Could you check a few things on this model? Use its own coordinates, in mm. Round coordinates to 2 decimals unless told otherwise and drop trailing zeros. Loops run counter-clockwise (first coordinate to the right, second up) from the corner with the lowest first, then second, coordinate; pieces in that order, holes last.
Autodesk Inventor part; units mm, degrees
ref_plane "YZ Plane" through (0, 0, 0) normal (1, 0, 0) x (0, 1, 0)
ref_plane "XZ Plane" through (0, 0, 0) normal (0, 1, 0) x (-1, 0, 0)
ref_plane "XY Plane" through (0, 0, 0) normal (0, 0, 1) x (1, 0, 0)
sketch "Sketch1" plane through (0, 0, 0) normal (0, 1, 0) x (-1, 0, 0)
  line L0 (12.5, -12.5) -> (-12.5, -12.5)
  line L1 (-12.5, -12.5) -> (-12.5, 12.5)
  line L2 (-12.5, 12.5) -> (12.5, 12.5)
  line L3 (12.5, 12.5) -> (12.5, -12.5)
  line L4 (12.5, -12.5) -> (-12.5, 12.5) construction
  line L5 (-12.5, -12.5) -> (12.5, 12.5) construction
  point P0 (0, 0)
  dimension "d0" = 25
  dimension "d1" = 25
extrude "Extrusion1" add sketch "Sketch1" along normal blind 2
sketch "Sketch2" plane through (0, 0, 0) normal (0, -1, 0) x (1, 0, 0)
  line L0 (-12.5, -12.5) -> (-12.5, 12.5) construction
  line L1 (-12.5, 12.5) -> (0, 0) construction
  line L2 (-12.5, 0) -> (0, 12.5) construction
  line L3 (-12.5, 12.5) -> (12.5, 12.5) construction
  circle A0 centre (-6.25, 6.25) radius 1.5
  line L4 (0, 12.5) -> (0, 0) construction
  line L5 (0, 0) -> (-12.5, 0) construction
  circle A1 centre (6.25, 6.25) radius 1.5
  circle A2 centre (-6.25, -6.25) radius 1.5
  circle A3 centre (6.25, -6.25) radius 1.5
  dimension "d4" = 3
extrude "Extrusion2" cut sketch "Sketch2" against normal blind 1
equation "\"d0\" = 0.125 * chessboard_length"
equation "\"d1\" = 0.125 * chessboard_width"
equation "\"d2\" = square_thickness"
equation "\"d4\" = peg_diameter"
equation "\"d5\" = peg_height"
equation "\"square_thickness\" = 2"
properties part number "White Square" material "ABS Plastic"
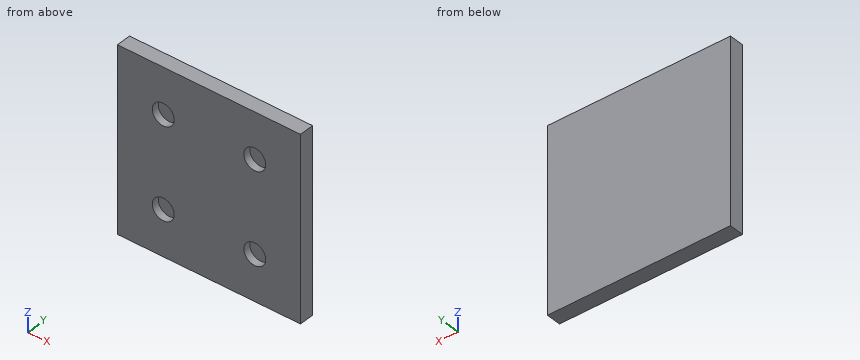
Item 1: Will these pins go through, and if not, where does the flat tip stop? pin 1 (0.9 mm diameter, centred on x = 6.5, z = 5.5, fed in from -Y); pin 2 (1.5 mm diameter, centred on x = -6.5, z = -5.5, fed in from -Y).
Results list:
pin 1: stops at y = 1
pin 2: stops at y = 0
Item 2: If I drill on line 1 along Z through (x, y) = (-6.25, 0.55); line 2 along X through (y, z) = (0.5, -5.25); line 3 along X through (y, z) = (0.3, -5.75), over which ranges is the centre line in solid material (lowest first)?
Results list:
line 1: z = -12.5 to -7.75, -4.75 to 4.75, 7.75 to 12.5
line 2: x = -12.5 to -7.37, -5.13 to 5.13, 7.37 to 12.5
line 3: x = -12.5 to -7.66, -4.84 to 4.84, 7.66 to 12.5
Item 3: If we section it at C-C, the plane x = -6.25: Please give me the cut outline in (y, z), then the cut area to 3 significant figures.
Results list:
outline: (0, -12.5) - (2, -12.5) - (2, 12.5) - (0, 12.5) - (0, 7.75) - (1, 7.75) - (1, 4.75) - (0, 4.75) - (0, -4.75) - (1, -4.75) - (1, -7.75) - (0, -7.75) - close
area: 44.0 mm2
Item 4: If we section it at B-B, the plane z = -6.25: Please give me the cut outline in (x, y), then the cut area to 3 significant figures.
Results list:
outline: (-12.5, 0) - (-7.75, 0) - (-7.75, 1) - (-4.75, 1) - (-4.75, 0) - (4.75, 0) - (4.75, 1) - (7.75, 1) - (7.75, 0) - (12.5, 0) - (12.5, 2) - (-12.5, 2) - close
area: 44.0 mm2
Item 5: If we section it at A-A, the plane y = 0.55: Please give me the cut outline in (x, z), then the cut area to 3 significant figures.
Results list:
outline: (-12.5, -12.5) - (12.5, -12.5) - (12.5, 12.5) - (-12.5, 12.5) - close; hole circle Ø3 at (-6.25, -6.25); hole circle Ø3 at (-6.25, 6.25); hole circle Ø3 at (6.25, -6.25); hole circle Ø3 at (6.25, 6.25)
area: 597 mm2
